Work out the finished part from the listing and answer in its coordinate system (mm). Give positions to 0.01 mm unless a question says otherwise; leave off trailing zeros. Loops run counter-clockwise (first coordinate to the right, second up) from the corner with the lowest first, then second, coordinate; pieces in that order, holes last. Notation, with made-up numbers: (-11.5, -35.5) - (22.5, -35.5) arc R7 cw to (22.5, -28.5) - close; hole circle Ø1 at (42, 51). An arc over 180 degrees is marked (long way). Use CSV: the item, a comma, the result in double quotes.
from build123d import *

# Parameters (mm, degrees)
F0_W     = 50.8
F0_H     = 508
F0_H_2   = 50.8
F0_R     = 9.525
F1_DEPTH = 19.05


with BuildPart() as f1:
    # F0 (on Top) → F1 (new body)
    with BuildSketch(Plane.XY):
        with Locations((25.4, 254)):
            Rectangle(F0_W, F0_H)
        with Locations((25.4, -25.4)):
            Rectangle(F0_W, F0_H_2)
        with Locations((25.4, -25.4)):
            Circle(F0_R, mode=Mode.SUBTRACT)
    extrude(amount=F1_DEPTH)


solid = f1.part
Item 1: A cutting plane is placed at B-B on x = 25.4. Determine the outline of the cut face in (y, z) (3 decimals), and give its area (3 significant figures).
Determined:
outline,"(-50.8, 0) - (-34.925, 0) - (-34.925, 19.05) - (-50.8, 19.05) - close; (-15.875, 0) - (508, 0) - (508, 19.05) - (-15.875, 19.05) - close"
area,"10,300 mm²"
Item 2: The mould has two halves that part along Y. Classify faces 1 (the flat face through (25, 233, 0)), 2 (the cylindrical face through (15.884, -24.981, 9.392)), 3 (the flat face through (25, 508, 9)), 4 (the flat face through (25, -50.8, 9)): pulls with the +Y half, pulls with the -Y half, needs draft (parallel to the pull), parting line crosses it, or undercut.
Determined:
face 1,"needs draft"
face 2,"undercut"
face 3,"pulls with the +Y half"
face 4,"pulls with the -Y half"
Item 3: Given P1, Ø17, axis at x = 25.4, y = -25.4, coming from the +Z side, flat-ended and moving along its own axis, determine where the tip first touches the part or whether it passes through.
Determined:
P1,"passes through"
Item 4: Find the intervals of material crossed by line 1 (Y direction, x = 24, z = 14); line 2 (Y direction, x = 25.4, z = 7) (3 decimals); line 3 (X direction, y = -24.5, z = 10), in increasing order.
Determined:
line 1,"y = -50.8 to -34.82, -15.98 to 508"
line 2,"y = -50.8 to -34.925, -15.875 to 508"
line 3,"x = 0 to 15.92, 34.88 to 50.8"
Item 5: A cutting plane is placed at A-A on y = -25.4. Determine the outline of the cut face in (x, z) (3 decimals), and give its area (3 significant figures).
Determined:
outline,"(0, 0) - (15.875, 0) - (15.875, 19.05) - (0, 19.05) - close; (34.925, 0) - (50.8, 0) - (50.8, 19.05) - (34.925, 19.05) - close"
area,"605 mm²"
